Geometry check sheet. Reference: the model listing, model coordinates, mm. A direction names the side the tool comes from. Give positions to 0.01 mm unless a question says otherwise; leave off trailing zeros. Write each loop counter-clockwise with the first axis right and the second up, starting at its lowest first coordinate (ties: lowest second). Pieces come first, ordered by that corner, then holes. Notation, with made-up numbers: (68.25, 83.5) -> (94.25, 83.5) arc R18 ccw to (94.25, 96.5) -> close; hole circle Ø11 at (2.5, 64). An arc over 180 degrees is marked (long way). Write item = value, one per line. Start each with the question number.
1. Cross-section at D-D, the plane x = -5.5. Record the cut outline in (y, z), plus the area to 3 significant figures.
2. Thickness scan on line 1 along Y through (x, z) = (-14, 3); line 2 along X through (y, z) = (-59.5, 10.5); line 3 along Y through (x, z) = (6.5, 11). Record the ranges inside material, lowest first.
3. Mould release check, pull along X, two halves, no side actions. Record for faces 1 (the flat face through (14, -30, 6)), 2 (the flat face through (49, -44, 23)), 3 (the flat face through (14, -31, 0)), 4 (the flat face through (-21, -43, 23)): pulls with the +X half, pulls with the -X half, needs draft (parallel to the pull), parting line crosses it, or undercut.
4. Cross-section at C-C, the plane y = -25.5. Record the cut outline in (x, z), plus the area to 3 significant figures.
5. Cross-section at A-A, the plane x = -14. Record the cut outline in (y, z), plus the area to 3 significant figures.
6. Set-up check for faces 5 (the flat face through (48, -7.141, 16)), 6 (the flat face through (-19, -44, 26)), 7 (the cylindrical face through (40.82, 0.94, 2.96)): record each of +Z, -Z, +X, -X, +Y, -Y from which the full face is reachable in a straight line by a thin tool's end or side.
7. Depth check by flat-ended pin: P1, Ø5, axis at x = 35.5, z = 17.5, coming from the +Y side; P2, Ø1.6, axis at x = -19.5, z = 17, coming from the +Y side; P3, Ø1.5, axis at x = -6, y = -60, coming from the +Z side. Enter the tip coordinate at first touch or a pass-through.
8. Cross-section at B-B, the plane z = 19.5. Record the cut outline in (x, y).
```python
from build123d import *

# Parameters (mm, degrees)
SKETCH_1_W          = 70
SKETCH_1_H          = 100
SKETCH_1_R          = 1.6
EXTRUDE_1_DEPTH     = 6
EXTRUDE_2_DEPTH     = 40
CUT_EXTRUDE_1_DEPTH = 71


with BuildPart() as part:
    # 草图1 → 凸台-拉伸1 (new body)
    with BuildSketch(Plane.XY):
        with Locations((14, -32.141025641)):
            Rectangle(SKETCH_1_W, SKETCH_1_H)
        with Locations((-14, -0.141025641)):
            Circle(SKETCH_1_R, mode=Mode.SUBTRACT)
        with Locations((42, -0.141025641)):
            Circle(SKETCH_1_R, mode=Mode.SUBTRACT)
    extrude(amount=EXTRUDE_1_DEPTH)

    # 草图2 → 凸台-拉伸2 (add)
    with BuildSketch(Plane.XY.offset(6)):
        Polygon((-19, -7.141025641), (-21, -7.141025641), (-21, -80.141025641), (-21, -82.141025641), (-18.055692248, -82.141025641), (46.014859647, -82.141025641), (49, -82.141025641), (49, -79.477981724), (49, -7.141025641), (47, -7.141025641), (47, -80.141025641), (-19, -80.141025641), align=None)
    extrude(amount=EXTRUDE_2_DEPTH)

    # 草图3 → 切除-拉伸1 (cut, through all)
    with BuildSketch(Plane.ZY.offset(21)):
        Polygon((26, -7.141025641), (46, -37.141025641), (46, -7.141025641), align=None)
    extrude(amount=-CUT_EXTRUDE_1_DEPTH, mode=Mode.SUBTRACT)


solid = part.part
```
Answers:
q1.outline = (-82.14, 0) -> (17.86, 0) -> (17.86, 6) -> (-80.14, 6) -> (-80.14, 46) -> (-82.14, 46) -> close
q1.area = 680 mm^2
q2.line_1 = -82.14 to -1.74, 1.46 to 17.86
q2.line_2 = -21 to -19, 47 to 49
q2.line_3 = -82.14 to -80.14
q3.face_1 = undercut
q3.face_2 = pulls with the +X half
q3.face_3 = needs draft
q3.face_4 = pulls with the -X half
q4.outline = (-21, 0) -> (49, 0) -> (49, 38.24) -> (47, 38.24) -> (47, 6) -> (-19, 6) -> (-19, 38.24) -> (-21, 38.24) -> close
q4.area = 549 mm^2
q5.outline = (-82.14, 0) -> (-1.74, 0) -> (-1.74, 6) -> (-80.14, 6) -> (-80.14, 46) -> (-82.14, 46) -> close; (1.46, 0) -> (17.86, 0) -> (17.86, 6) -> (1.46, 6) -> close
q5.area = 661 mm^2
q6.face_5 = +Z, +X, -X, +Y
q6.face_6 = +Z, +Y
q6.face_7 = +Z, -Z
q7.P1 = -80.14
q7.P2 = -7.14
q7.P3 = 6
q8.outline = (-21, -82.14) -> (49, -82.14) -> (49, -7.14) -> (47, -7.14) -> (47, -80.14) -> (-19, -80.14) -> (-19, -7.14) -> (-21, -7.14) -> close
